from build123d import *

# Parameters (mm, degrees)
SKETCH2_R           = 5
BOSS_EXTRUDE1_DEPTH = 7
SKETCH3_R           = 6.75
BOSS_EXTRUDE2_DEPTH = 1.25
BOSS_EXTRUDE3_START = -7
SKETCH3_2_R         = 6.75
BOSS_EXTRUDE3_DEPTH = 1.25
SKETCH4_R           = 3.5
CUT_EXTRUDE1_DEPTH  = 3
SKETCH5_R           = 3.5
CUT_EXTRUDE2_DEPTH  = 3
SKETCH6_R           = 2
CUT_EXTRUDE3_DEPTH  = 7.5
CHAMFER1_SIZE       = 0.5


with BuildPart() as part:
    # Sketch2 → Boss-Extrude1 (new body)
    with BuildSketch(Plane(origin=(0, 0, 0), x_dir=(1, 0, 0), z_dir=(0, 1, 0))):
        Circle(SKETCH2_R)
    extrude(amount=BOSS_EXTRUDE1_DEPTH)

    # Sketch3 → Boss-Extrude2 (add)
    with BuildSketch(Plane(origin=(0, 7, 0), x_dir=(1, 0, 0), z_dir=(0, 1, 0))):
        Circle(SKETCH3_R)
    extrude(amount=BOSS_EXTRUDE2_DEPTH)

    # Sketch3<2> → Boss-Extrude3 (add)
    with BuildSketch(Plane(origin=(0, 7, 0), x_dir=(1, 0, 0), z_dir=(0, 1, 0)).offset(BOSS_EXTRUDE3_START)):
        Circle(SKETCH3_2_R)
    extrude(amount=-BOSS_EXTRUDE3_DEPTH)

    # Sketch4 → Cut-Extrude1 (cut)
    with BuildSketch(Plane.XZ.offset(1.25)):
        Circle(SKETCH4_R)
    extrude(amount=-CUT_EXTRUDE1_DEPTH, mode=Mode.SUBTRACT)

    # Sketch5 → Cut-Extrude2 (cut)
    with BuildSketch(Plane(origin=(0, 8.25, 0), x_dir=(1, 0, 0), z_dir=(0, 1, 0))):
        Circle(SKETCH5_R)
    extrude(amount=-CUT_EXTRUDE2_DEPTH, mode=Mode.SUBTRACT)

    # Sketch6 → Cut-Extrude3 (cut, through all)
    with BuildSketch(Plane(origin=(0, 5.25, 0), x_dir=(1, 0, 0), z_dir=(0, 1, 0))):
        Circle(SKETCH6_R)
    extrude(amount=-CUT_EXTRUDE3_DEPTH, mode=Mode.SUBTRACT)

    # Chamfer1
    chamfer1_edges = [part.edges().sort_by_distance(p)[0] for p in [
        (-3.5, -1.25, 0),
        (-3.5, 8.25, 0),
    ]]
    chamfer(chamfer1_edges, length=CHAMFER1_SIZE)


solid = part.part
Verification items for the finished model (mm, model axes). A direction names the side the tool comes from. Round coordinates to 2 decimals unless told otherwise and drop trailing zeros. Loops run counter-clockwise (first coordinate to the right, second up) from the corner with the lowest first, then second, coordinate; pieces in that order, holes last. Notation, with made-up numbers: M 53,30 L 66,30 A22 cw 66,62 Z; hole C -9.75,-5 d4. An arc over 180 degrees is marked long. Write each question's results on one line, items separated by ' | '.
1) Section check C-C on y = 6. Record the boundary of the cut face in (x, z), then the cut area to 3 significant figures.
Checks:
outline: C 0,0 d10; hole C 0,0 d7 | area: 40.1 mm2
2) Section check A-A on x = 0. Record the boundary of the cut face in (y, z).
Checks:
outline: M -1.25,-6.75 L 0,-6.75 L 0,-5 L 7,-5 L 7,-6.75 L 8.25,-6.75 L 8.25,-4 L 7.75,-3.5 L 5.25,-3.5 L 5.25,-2 L 1.75,-2 L 1.75,-3.5 L -0.75,-3.5 L -1.25,-4 Z; M -1.25,4 L -0.75,3.5 L 1.75,3.5 L 1.75,2 L 5.25,2 L 5.25,3.5 L 7.75,3.5 L 8.25,4 L 8.25,6.75 L 7,6.75 L 7,5 L 0,5 L 0,6.75 L -1.25,6.75 Z
3) Gauge pin test, flat ends, axial feed: P1, Ø4, axis at x = 2, z = -2, coming from the +Y side; P2, Ø4, axis at x = -0.5, z = 1, coming from the +Y side; P3, Ø2, axis at x = 3, y = 6.5, coming from the +Z side; P4, Ø6.5, axis at x = 0, z = 0, coming from the -Y side. Record the tip position at first contact, or that the pin passes through.
Checks:
P1: stops at y = 8.25 | P2: stops at y = 5.25 | P3: stops at z = 6.4 | P4: stops at y = 1.75
4) Scan lines: L1, parallel to Z at x = 0, y = 3.95; L2, parallel to X at y = 6.25, z = 0; L3, parallel to Y at x = -3.25, z = 5. Record each from-to range of solid material in increasing order. Write a range as from..to.
Checks:
L1: z = -5..-2, 2..5 | L2: x = -5..-3.5, 3.5..5 | L3: y = -1.25..0, 7..8.25
5) Section check D-D on y = 4. Record the boundary of the cut face in (x, z).
Checks:
outline: C 0,0 d10; hole C 0,0 d4
6) Mould release check, pull along Y, two halves, no side actions. Record for faces 5 (the flat face through (3, 8.25, 3)), 6 (the cylindrical face through (-1.08, 3.45, 4.88)), 7 (the flat face through (3, -1.25, 3)): released by +Y, released by -Y, zero draft, split by the parting line, or undercut.
Checks:
face 5: released by +Y | face 6: undercut | face 7: released by -Y
7) Section check B-B on z = 0. Record the boundary of the cut face in (x, y).
Checks:
outline: M -6.75,-1.25 L -4,-1.25 L -3.5,-0.75 L -3.5,1.75 L -2,1.75 L -2,5.25 L -3.5,5.25 L -3.5,7.75 L -4,8.25 L -6.75,8.25 L -6.75,7 L -5,7 L -5,0 L -6.75,0 Z; M 2,1.75 L 3.5,1.75 L 3.5,-0.75 L 4,-1.25 L 6.75,-1.25 L 6.75,0 L 5,0 L 5,7 L 6.75,7 L 6.75,8.25 L 4,8.25 L 3.5,7.75 L 3.5,5.25 L 2,5.25 Z
8) Access from +Z, -Z, +X, -X, +Y, -Y to the whole of each face (thin tool, end or side, straight path). Record for faces 1 (the cylindrical face through (3.233, 0.482, -1.341)), 2 (the cylindrical face through (-1.46, -0.62, 6.59)), 3 (the flat face through (-5, 7, 2)), 4 (the flat face through (2, 5.25, 2)).
Checks:
face 1: -Y | face 2: +Y, -Y | face 3: none | face 4: +Y
